from build123d import *

# Parameters (mm, degrees)
SKETCH1_W           = 250
SKETCH1_H           = 150
SKETCH1_R           = 4.1
BOSS_EXTRUDE1_DEPTH = 6
SKETCH2_W           = 62
SKETCH2_H           = 31
CUT_EXTRUDE1_DEPTH  = 2
SKETCH3_R           = 17
SKETCH3_R_2         = 2.125
CUT_EXTRUDE3_DEPTH  = 29


with BuildPart() as part:
    # Sketch1 → Boss-Extrude1 (new body)
    with BuildSketch(Plane(origin=(0, 0, 0), x_dir=(1, 0, 0), z_dir=(0, 1, 0))):
        Rectangle(SKETCH1_W, SKETCH1_H)
        with Locations((15, -20.5)):
            Circle(SKETCH1_R, mode=Mode.SUBTRACT)
        with Locations((-15, -20.5)):
            Circle(SKETCH1_R, mode=Mode.SUBTRACT)
    extrude(amount=BOSS_EXTRUDE1_DEPTH)

    # Sketch2 → Cut-Extrude1 (cut)
    with BuildSketch(Plane(origin=(0, 6, 0), x_dir=(1, 0, 0), z_dir=(0, 1, 0))):
        with Locations((0, -20.5)):
            Rectangle(SKETCH2_W, SKETCH2_H)
    extrude(amount=-CUT_EXTRUDE1_DEPTH, mode=Mode.SUBTRACT)

    # Sketch3 → Cut-Extrude3 (cut)
    with BuildSketch(Plane(origin=(0, 6, 0), x_dir=(1, 0, 0), z_dir=(0, 1, 0))):
        Polygon((22.5, 20), (-22.5, 20), (-22.5, -5), (0, -5), (22.5, -5), align=None)
        with Locations((-85, 0.222388038)):
            Circle(SKETCH3_R)
        with Locations((85, 0.222388038)):
            Circle(SKETCH3_R)
        with Locations((-97, 18.222388038)):
            Circle(SKETCH3_R_2)
        with Locations((-97, -17.777611962)):
            Circle(SKETCH3_R_2)
        with Locations((-73, -17.777611962)):
            Circle(SKETCH3_R_2)
        with Locations((-73, 18.222388038)):
            Circle(SKETCH3_R_2)
        with Locations((73, -17.777611962)):
            Circle(SKETCH3_R_2)
        with Locations((97, -17.777611962)):
            Circle(SKETCH3_R_2)
        with Locations((97, 18.222388038)):
            Circle(SKETCH3_R_2)
        with Locations((73, 18.222388038)):
            Circle(SKETCH3_R_2)
    extrude(amount=-CUT_EXTRUDE3_DEPTH, mode=Mode.SUBTRACT)


solid = part.part
Design review of the part built by this model. Coordinates are the model's own, in mm. A direction names the side the tool comes from. Coordinates: 2 decimals unless noted, no trailing zeros. Order: outer loops, then holes, each group sorted by start corner. A loop starts at its lowest first (then second) coordinate and runs counter-clockwise, first axis right, second up.
Item 1: Take a section at C-C, the plane z = -3. Write out the cut boundary in (x, y).
Item 2: Take a section at D-D, the plane y = 5.1. Count the separate pieces of the cut face and the enclosed holes in it, then the cut area to 3 significant figures.
Item 3: For faces 4 (the flat face through (22.5, 3, -7)), 5 (the flat face through (-30, 6, -1)), 6 (the flat face through (0, 4, 20)), list the 3-axis set-ups (+Z, -Z, +X, -X, +Y, -Y) from which the entire face can be reached by the end or side of a thin tool; tool diameter is ignored.
Item 4: For line 1 (X direction, y = 2.4, z = 20.5); line 2 (X direction, y = 1.15, z = -18); line 3 (Z direction, x = -73, y = 2.6), list the stretches that pass through material, from the lowest coordinate up.
Item 5: Take a section at B-B, the plane x = -85. Write out the cut boundary in (y, z), then the cut area to 3 significant figures.
Item 6: For pin 1 Ø1 at (x, z) = (-15.5, 6.5) entering from +Y, flat-tipped, find the tip position at first contact; note if it passes through.
Item 7: Take a section at A-A, the plane x = 15. Write out the cut boundary in (y, z), then the cut area to 3 significant figures.
Item 8: The part is to be moulded in two halves that separate along Z. For faces 1 (the flat face through (-2, 3, -75)), 2 (the flat face through (-22.5, 3, -8)), 3 (the flat face through (-125, 3, 1)), say which applies: pulls with the +Z half, pulls with the -Z half, needs draft (parallel to the pull), parting line crosses it, or undercut.
The answers:
1. outline: (-125, 0) - (-101.77, 0) - (-101.77, 6) - (-125, 6) - close; (-68.23, 0) - (-22.5, 0) - (-22.5, 6) - (-68.23, 6) - close; (22.5, 0) - (68.23, 0) - (68.23, 6) - (22.5, 6) - close; (101.77, 0) - (125, 0) - (125, 6) - (101.77, 6) - close
2. separate pieces: 1
2. enclosed holes: 11
2. area: 32,500 mm2
3. face 4: +Y, -Y
3. face 5: +Z, -Z, +X, -X, +Y
3. face 6: +Y
4. line 1: x = -125 to -19.1, -10.9 to 10.9, 19.1 to 125
4. line 2: x = -125 to -99.11, -94.89 to -75.11, -70.89 to -22.5, 22.5 to 70.89, 75.11 to 94.89, 99.11 to 125
4. line 3: z = -75 to -20.35, -16.1 to -12.26, 11.82 to 15.65, 19.9 to 75
5. outline: (0, -75) - (6, -75) - (6, -17.22) - (0, -17.22) - close; (0, 16.78) - (6, 16.78) - (6, 75) - (0, 75) - close
5. area: 696 mm2
6. pin 1: stops at y = 4
7. outline: (0, -75) - (6, -75) - (6, -20) - (0, -20) - close; (0, 5) - (4, 5) - (4, 16.4) - (0, 16.4) - close; (0, 24.6) - (4, 24.6) - (4, 36) - (6, 36) - (6, 75) - (0, 75) - close
7. area: 655 mm2
8. face 1: pulls with the -Z half
8. face 2: undercut
8. face 3: needs draft
